Geometry: see drawing. Coordinates: mm, zero at the bounding-box minimum. Give positions to 0.01 mm unless a question says otherwise; leave off trailing zeros. Loops run counter-clockwise (first coordinate to the right, second up) from the corner with the lowest first, then second, coordinate; pieces in that order, holes last. Notation, with made-up numbers: (-4.75, 25.5) -> (13.25, 25.5) arc R15 ccw to (13.25, 50.5) -> close; hole circle Ø2 at (51.25, 59). An arc over 180 degrees is marked (long way). Return JSON: item names as keys, results as strings. Group by question number.
(1) Cut plane C-C on z = 179.5. Return loops of the section in (x, y).
(2) Draft query along Z for the marked faces 1, 2, 3 and 4. Return one class per face: released by +Z, released by -Z, zero draft, split by the parting line, or undercut.
(3) Ray query, line 1 (Z direction, x = 66, y = 18); line 2 (Y direction, x = 15.5, z = 154); line 3 (Z direction, x = 48, y = 3.5). Return the intervals inside material, ascending. Write a range as from..to.
(4) Cut plane A-A on y = 37.5. Return loops of the section in (x, z), then the cut area to 3 significant figures.
(5) Cut plane B-B on x = 23. Return loops of the section in (y, z).
(6) Pin query (flat end, axial travel): pin 1 (2 mm diameter, centred on x = 63.5, z = 25.5, fed in from +Y); pin 2 (3 mm diameter, centred on x = 100.5, y = 4, fed in from -Z). Return the tip coordinate at first contact, or that it passes through.
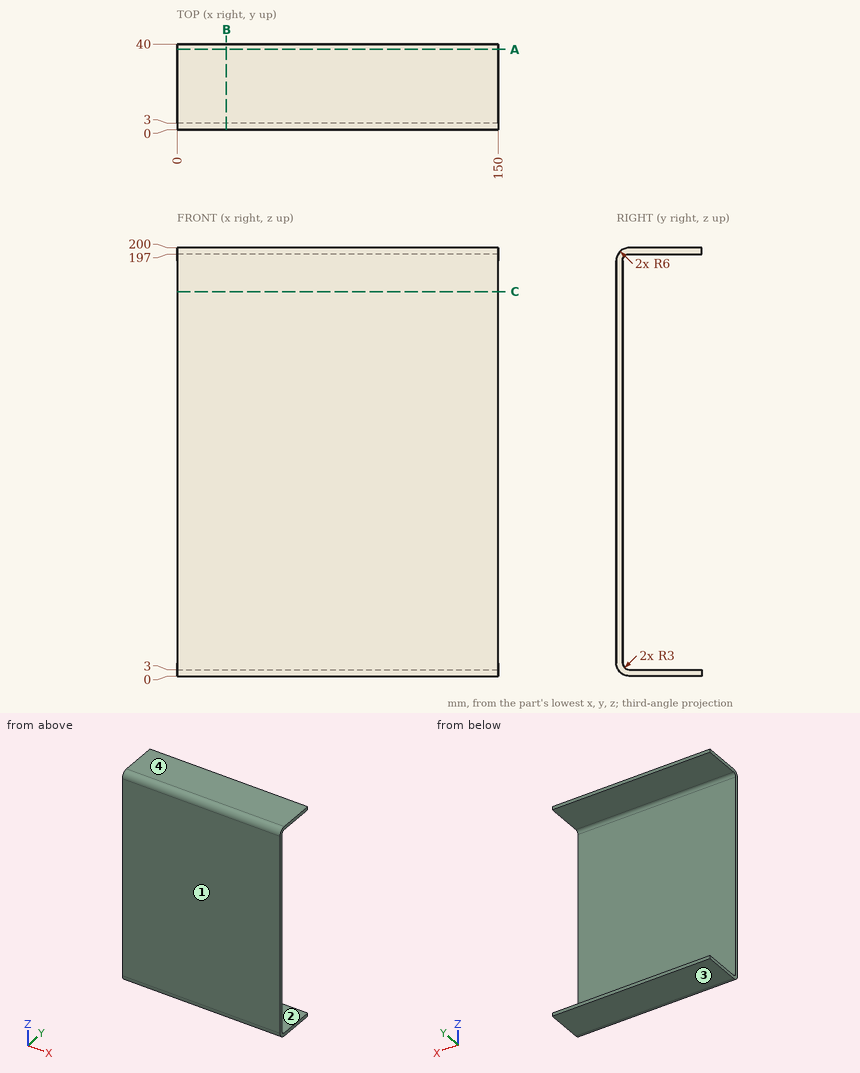
Answers:
{
 "1": {"outline": "(0, 0) -> (150, 0) -> (150, 3) -> (0, 3) -> close"},
 "2": {"face 1": "zero draft", "face 2": "undercut", "face 3": "released by -Z", "face 4": "released by +Z"},
 "3": {"line 1": "0..3, 197..200", "line 2": "0..3", "line 3": "0.55..4.34, 195.66..199.45"},
 "4": {"outline": "(0, 0) -> (150, 0) -> (150, 3) -> (0, 3) -> close; (0, 197) -> (150, 197) -> (150, 200) -> (0, 200) -> close", "area": "900 mm²"},
 "5": {"outline": "(0, 6) arc R6 ccw to (6, 0) -> (40, 0) -> (40, 3) -> (6, 3) arc R3 cw to (3, 6) -> (3, 194) arc R3 cw to (6, 197) -> (40, 197) -> (40, 200) -> (6, 200) arc R6 ccw to (0, 194) -> close"},
 "6": {"pin 1": "y = 3", "pin 2": "z = 0.02"}
}
